Work out the finished part from the listing and answer in its coordinate system (mm). A direction names the side the tool comes from. Give positions to 0.01 mm unless a question says otherwise; leave off trailing zeros. Loops run counter-clockwise (first coordinate to the right, second up) from the corner with the lowest first, then second, coordinate; pieces in that order, holes last. Notation, with made-up numbers: (74, -31.75) - (91, -31.75) arc R29 cw to (91, -9.75) - close; hole circle Ø6 at (-15, 45.5). An arc over 180 degrees is marked (long way). One line per item, written item: value.
from build123d import *

# Parameters (mm, degrees)
SKETCH_1_R          = 3
SKETCH_1_R_2        = 1.5
EXTRUDE_1_DEPTH     = 4
SKETCH_3_R          = 13
CUT_EXTRUDE_2_DEPTH = 2


with BuildPart() as part:
    # 草图1 → 凸台-拉伸1 (new body)
    with BuildSketch(Plane.XY):
        with BuildLine():
            Line((1789.5396377, 1516.163703518), (1794.90094238, 1510.03649817))
            ThreePointArc((1794.90094238, 1510.03649817), (1795.919023617, 1509.280113251), (1797.158672464, 1509.012011993))
            Line((1797.158672464, 1509.012011993), (1805.574426245, 1509.012011993))
            ThreePointArc((1805.574426245, 1509.012011993), (1806.70688816, 1509.233967715), (1807.671779141, 1509.866991986))
            Line((1807.671779141, 1509.866991986), (1850.89472068, 1552.129423713))
            ThreePointArc((1850.89472068, 1552.129423713), (1851.562513231, 1553.110841273), (1851.797367784, 1554.274443721))
            Line((1851.797367784, 1554.274443721), (1851.797367784, 1565.749580266))
            ThreePointArc((1851.797367784, 1565.749580266), (1851.562513231, 1566.913182714), (1850.89472068, 1567.894600273))
            Line((1850.89472068, 1567.894600273), (1807.671779141, 1610.157032))
            ThreePointArc((1807.671779141, 1610.157032), (1806.70688816, 1610.790056271), (1805.574426245, 1611.012011993))
            Line((1805.574426245, 1611.012011993), (1797.158672464, 1611.012011993))
            ThreePointArc((1797.158672464, 1611.012011993), (1795.919023617, 1610.743910735), (1794.90094238, 1609.987525817))
            Line((1794.90094238, 1609.987525817), (1789.5396377, 1603.860320468))
            ThreePointArc((1789.5396377, 1603.860320468), (1788.989059552, 1602.939986664), (1788.797367784, 1601.884806645))
            Line((1788.797367784, 1601.884806645), (1788.797367784, 1518.139217341))
            ThreePointArc((1788.797367784, 1518.139217341), (1788.989059552, 1517.084037322), (1789.5396377, 1516.163703518))
        make_face()
        with Locations((1800.797367784, 1560.012011993)):
            Circle(SKETCH_1_R, mode=Mode.SUBTRACT)
        with Locations((1800.797367784, 1602.512011993)):
            Circle(SKETCH_1_R_2, mode=Mode.SUBTRACT)
        with Locations((1843.297367784, 1560.012011993)):
            Circle(SKETCH_1_R_2, mode=Mode.SUBTRACT)
        with Locations((1800.797367784, 1517.512011993)):
            Circle(SKETCH_1_R_2, mode=Mode.SUBTRACT)
        with BuildLine():
            ThreePointArc((1805.443255224, 1552.809308797), (1806.858027956, 1553.951351821), (1808.000070981, 1555.366124554))
            ThreePointArc((1808.000070981, 1555.366124554), (1807.55260939, 1557.43971519), (1805.479018754, 1556.992253599))
            ThreePointArc((1805.479018754, 1556.992253599), (1804.736707613, 1556.072672165), (1803.817126178, 1555.330361023))
            ThreePointArc((1803.817126178, 1555.330361023), (1803.369664588, 1553.256770387), (1805.443255224, 1552.809308797))
        make_face(mode=Mode.SUBTRACT)
        with BuildLine():
            ThreePointArc((1808.000070981, 1564.657899433), (1806.858027956, 1566.072672165), (1805.443255224, 1567.21471519))
            ThreePointArc((1805.443255224, 1567.21471519), (1803.369664588, 1566.767253599), (1803.817126178, 1564.693662963))
            ThreePointArc((1803.817126178, 1564.693662963), (1804.736707613, 1563.951351821), (1805.479018754, 1563.031770387))
            ThreePointArc((1805.479018754, 1563.031770387), (1807.55260939, 1562.584308797), (1808.000070981, 1564.657899433))
        make_face(mode=Mode.SUBTRACT)
        with BuildLine():
            ThreePointArc((1796.151480345, 1567.21471519), (1794.736707613, 1566.072672165), (1793.594664588, 1564.657899433))
            ThreePointArc((1793.594664588, 1564.657899433), (1794.042126178, 1562.584308797), (1796.115716814, 1563.031770387))
            ThreePointArc((1796.115716814, 1563.031770387), (1796.858027956, 1563.951351821), (1797.77760939, 1564.693662963))
            ThreePointArc((1797.77760939, 1564.693662963), (1798.225070981, 1566.767253599), (1796.151480345, 1567.21471519))
        make_face(mode=Mode.SUBTRACT)
        with BuildLine():
            ThreePointArc((1793.594664588, 1555.366124554), (1794.736707613, 1553.951351821), (1796.151480345, 1552.809308797))
            ThreePointArc((1796.151480345, 1552.809308797), (1798.225070981, 1553.256770387), (1797.77760939, 1555.330361023))
            ThreePointArc((1797.77760939, 1555.330361023), (1796.858027956, 1556.072672165), (1796.115716814, 1556.992253599))
            ThreePointArc((1796.115716814, 1556.992253599), (1794.042126178, 1557.43971519), (1793.594664588, 1555.366124554))
        make_face(mode=Mode.SUBTRACT)
    extrude(amount=EXTRUDE_1_DEPTH)

    # 草图3 → 切除-拉伸2 (cut)
    with BuildSketch(Plane(origin=(0, 0, 0), x_dir=(-1, 0, 0), z_dir=(0, 0, -1))):
        with Locations((-1800.797367784, 1560.012011993)):
            Circle(SKETCH_3_R)
    extrude(amount=-CUT_EXTRUDE_2_DEPTH, mode=Mode.SUBTRACT)


solid = part.part
1. Section C-C (y = 1550) is taken. Write down the section's boundary in (x, z), and give its area (3 significant figures).
Output:
outline: (1788.8, 0) - (1792.51, 0) - (1792.51, 2) - (1809.09, 2) - (1809.09, 0) - (1848.72, 0) - (1848.72, 4) - (1788.8, 4) - close
area: 207 mm²
2. Section B-B (z = 1) is taken. Write down the section's boundary in (x, y), and give its area (3 significant figures).
Output:
outline: (1788.8, 1518.14) arc R3 ccw to (1789.54, 1516.16) - (1794.9, 1510.04) arc R3 ccw to (1797.16, 1509.01) - (1805.57, 1509.01) arc R3 ccw to (1807.67, 1509.87) - (1850.89, 1552.13) arc R3 ccw to (1851.8, 1554.27) - (1851.8, 1565.75) arc R3 ccw to (1850.89, 1567.89) - (1807.67, 1610.16) arc R3 ccw to (1805.57, 1611.01) - (1797.16, 1611.01) arc R3 ccw to (1794.9, 1609.99) - (1789.54, 1603.86) arc R3 ccw to (1788.8, 1601.88) - (1788.8, 1565.01) arc R13 cw (long way) to (1788.8, 1555.01) - close; hole circle Ø3 at (1800.8, 1517.51); hole circle Ø3 at (1800.8, 1602.51); hole circle Ø3 at (1843.3, 1560.01)
area: 3,840 mm²
3. Flat-ended cylindrical pins translate along their axes: pin 1 Ø15.5 at (x, y) = (1800.8, 1560.01) entering from -Z; pin 2 Ø5 at (x, y) = (1819, 1584) entering from -Z; pin 3 Ø1.5 at (y, z) = (1573.5, 0.5) entering from +X. Find the tip coordinate at first contact, or state that the pin passes through.
Output:
pin 1: stops at z = 2
pin 2: stops at z = 0
pin 3: stops at x = 1845.93
4. Section A-A (x = 1811.5) is taken. Write down the section's boundary in (y, z).
Output:
outline: (1513.61, 0) - (1552.63, 0) - (1552.63, 2) - (1567.39, 2) - (1567.39, 0) - (1606.41, 0) - (1606.41, 4) - (1513.61, 4) - close
5. Section D-D (y = 1593) is taken. Write down the section's boundary in (x, z), and give its area (3 significant figures).
Output:
outline: (1788.8, 0) - (1825.22, 0) - (1825.22, 4) - (1788.8, 4) - close
area: 146 mm²
6. Find the intervals of material crossed by line 1 along X through (y, z) = (1560, 2.4); line 2 along Y through (x, z) = (1804, 2.45); line 3 along Y through (x, z) = (1793.5, 2.3), in increasing order.
Output:
line 1: x = 1788.8 to 1797.8, 1803.8 to 1841.8, 1844.8 to 1851.8
line 2: y = 1509.01 to 1552.71, 1555.45 to 1564.57, 1567.32 to 1611.01
line 3: y = 1511.64 to 1555.54, 1556.82 to 1563.2, 1564.49 to 1608.39
7. For faces 5 (the flat face through (1813, 1561, 4)), 6 (the flat face through (1801.5, 1563.1, 2)), 7 (the cylindrical face through (1806.84, 1553.933, 2.986)), determine the directions among +Z, -Z, +X, -X, +Y, -Y from which every point of the face is accessible in a straight line to the end or side of a thin tool.
Output:
face 5: +Z, +X, -X, +Y, -Y
face 6: -Z
face 7: +Z, -Z
8. The mould has two halves that part along Y. Classify faces 1 (the cylindrical face through (1802.23, 1602.96, 1.97)), 2 (the cylindrical face through (1798.24, 1566.74, 2.99)), 3 (the flat face through (1792.183, 1513.143, 1.972)), 4 (the flat face through (1801, 1611.012, 2)): released by +Y, released by -Y, zero draft, split by the parting line, or undercut.
Output:
face 1: undercut
face 2: undercut
face 3: released by -Y
face 4: released by +Y
